The drawing under review shows one solid part. Ordinate dimensions are in mm from its lowest x, y, z. Round coordinates to 2 decimals unless told otherwise and drop trailing zeros. Write each loop counter-clockwise with the first axis right and the second up, starting at its lowest first coordinate (ties: lowest second). Pieces come first, ordered by that corner, then holes. Notation, with made-up numbers: (56.5, -10) -> (109.5, -10) arc R19 cw to (109.5, 19) -> close; hole circle Ø9 at (4.5, -22.5). An arc over 180 degrees is marked (long way). Answer in a Markdown table with one row per item. Add a question column.
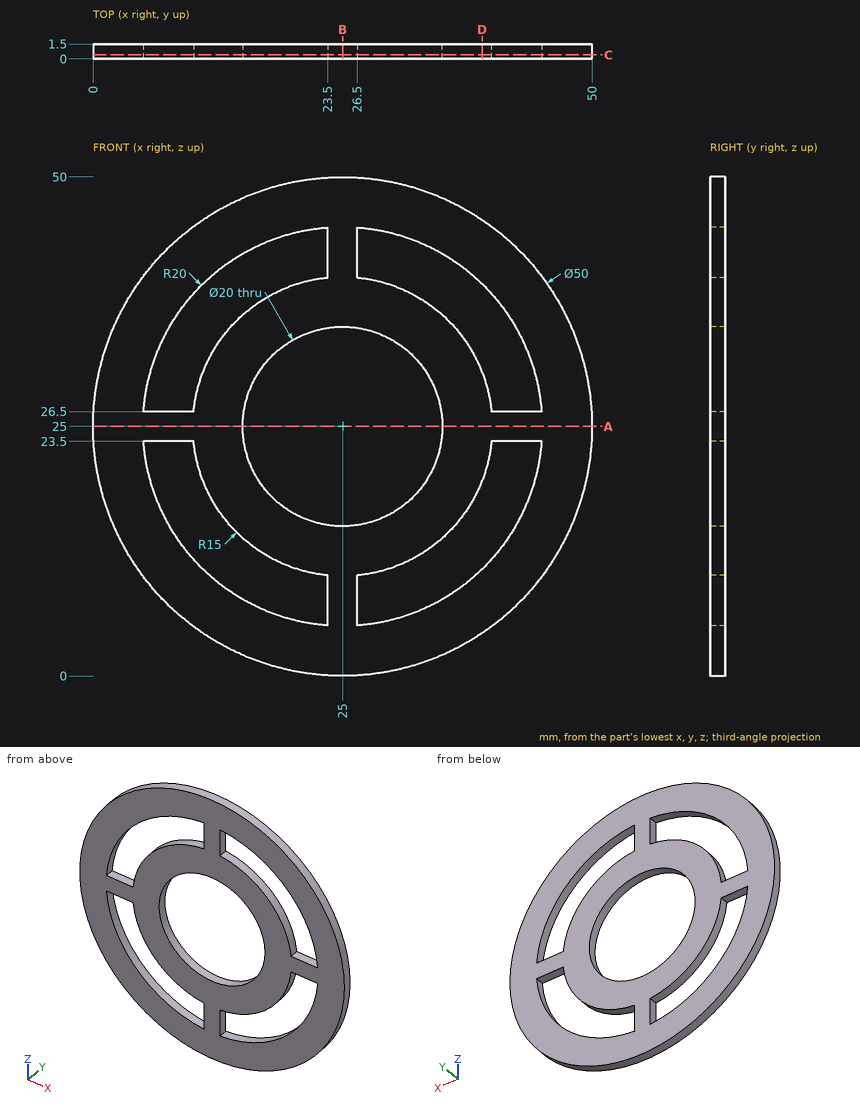
1. Insertion check: pin 1 Ø0.8 at (y, z) = (0.5, 8) entering from -X; pin 2 Ø10 at (x, z) = (15.5, 18.5) entering from -Y; pin 3 Ø0.8 at (x, y) = (7.5, 1) entering from -Z. Each pin has a flat end and moves straight along its axis. Give the tip position at first contact, or say it passes through.
2. Add section A-A on z = 25. Write out the cut boundary in (x, y), plus the area to 3 significant figures.
3. Add section B-B on x = 25. Write out the cut boundary in (y, z).
4. Add section D-D on x = 39. Write out the cut boundary in (y, z), plus the area to 3 significant figures.
5. Add section C-C on y = 0.4. Write out the cut boundary in (x, z).
6. For L1, parallel to Z at x = 25, y = 0.45; L2, parallel to X at y = 0.8, z = 29; L3, parallel to Z at x = 35.5, y = 1.45, list the stretches that pass through material, from the lowest coordinate up.
Filled in:
| question | item | result |
|---|---|---|
| 1 | pin 1 | x = 6.31 |
| 1 | pin 2 | y = 0 |
| 1 | pin 3 | z = 6.76 |
| 2 | outline | (0, 0) -> (15, 0) -> (15, 1.5) -> (0, 1.5) -> close; (35, 0) -> (50, 0) -> (50, 1.5) -> (35, 1.5) -> close |
| 2 | area | 45.0 mm² |
| 3 | outline | (0, 0) -> (1.5, 0) -> (1.5, 15) -> (0, 15) -> close; (0, 35) -> (1.5, 35) -> (1.5, 50) -> (0, 50) -> close |
| 4 | outline | (0, 4.29) -> (1.5, 4.29) -> (1.5, 10.72) -> (0, 10.72) -> close; (0, 19.61) -> (1.5, 19.61) -> (1.5, 30.39) -> (0, 30.39) -> close; (0, 39.28) -> (1.5, 39.28) -> (1.5, 45.71) -> (0, 45.71) -> close |
| 4 | area | 35.4 mm² |
| 5 | outline | circle Ø50 at (25, 25); hole (5.06, 23.5) arc R20 ccw to (23.5, 5.06) -> (23.5, 10.08) arc R15 cw to (10.08, 23.5) -> close; hole (5.06, 26.5) -> (10.08, 26.5) arc R15 cw to (23.5, 39.92) -> (23.5, 44.94) arc R20 ccw to start; hole circle Ø20 at (25, 25); hole (26.5, 5.06) arc R20 ccw to (44.94, 23.5) -> (39.92, 23.5) arc R15 cw to (26.5, 10.08) -> close; hole (26.5, 39.92) arc R15 cw to (39.92, 26.5) -> (44.94, 26.5) arc R20 ccw to (26.5, 44.94) -> close |
| 6 | L1 | 0 to 15, 35 to 50 |
| 6 | L2 | 0.32 to 5.4, 10.54 to 15.83, 34.17 to 39.46, 44.6 to 49.68 |
| 6 | L3 | 2.31 to 7.98, 14.29 to 35.71, 42.02 to 47.69 |
